```python
from build123d import *

# Parameters (mm, degrees)
F0_W      = 19
F0_H      = 30
F1_DEPTH  = 5
F3_DEPTH  = 3
F4_R      = 1
F4_R_2    = 0.895507
F5_DEPTH  = 25
F6_DEPTH  = 25
F7_W      = 43.592543
F7_H      = 48.578868
F8_DEPTH  = 2
F9_W      = 52.903849
F9_H      = 60.980772
F10_DEPTH = 1
F11_DEPTH = 25


with BuildPart() as f1:
    # F0 (on Front) → F1 (new body)
    with BuildSketch(Plane.XZ):
        Rectangle(F0_W, F0_H)
    extrude(amount=F1_DEPTH)

    # F2 (on face) → F3 (cut)
    with BuildSketch(Plane.XZ.offset(5)):
        with BuildLine():
            Line((-3, 0), (-3, -9))
            ThreePointArc((-3, -9), (0, -12), (3, -9))
            Line((3, -9), (3, 0))
            ThreePointArc((3, 0), (0, 2.961188), (-3, 0))
        make_face()
    extrude(amount=-F3_DEPTH, mode=Mode.SUBTRACT)

    # F4 (on face) → F5 (cut)
    with BuildSketch(Plane.XZ.offset(2)):
        with Locations((-6.5, 12)):
            Circle(F4_R)
        with Locations((6.5, 12)):
            Circle(F4_R)
        with Locations((6.5, -12)):
            Circle(F4_R)
        with Locations((-6.5, -12)):
            Circle(F4_R)
        with Locations((-6.5, 0)):
            Circle(F4_R)
        with Locations((6.5, 0)):
            Circle(F4_R_2)
    extrude(amount=-F5_DEPTH, mode=Mode.SUBTRACT)

    # F4 (on face) → F6 (cut)
    with BuildSketch(Plane.XZ.offset(2)):
        with Locations((-6.5, 12)):
            Circle(F4_R)
        with Locations((6.5, 12)):
            Circle(F4_R)
        with Locations((6.5, -12)):
            Circle(F4_R)
        with Locations((-6.5, -12)):
            Circle(F4_R)
        with Locations((-6.5, 0)):
            Circle(F4_R)
        with Locations((6.5, 0)):
            Circle(F4_R_2)
    extrude(amount=F6_DEPTH, mode=Mode.SUBTRACT)

    # F7 (on face) → F8 (cut)
    with BuildSketch(Plane.XZ.offset(5)):
        with Locations((0.917289, -2.192111)):
            Rectangle(F7_W, F7_H)
    extrude(amount=-F8_DEPTH, mode=Mode.SUBTRACT)

    # F9 (on face) → F10 (cut)
    with BuildSketch(Plane(origin=(0, 0, 0), x_dir=(-1, 0, 0), z_dir=(0, 1, 0))):
        with Locations((0.067309, -0.875001)):
            Rectangle(F9_W, F9_H)
    extrude(amount=-F10_DEPTH, mode=Mode.SUBTRACT)

    # F2 (on face) → F11 (cut)
    with BuildSketch(Plane.XZ.offset(5)):
        with BuildLine():
            Line((-3, 0), (-3, -9))
            ThreePointArc((-3, -9), (0, -12), (3, -9))
            Line((3, -9), (3, 0))
            ThreePointArc((3, 0), (0, 2.961188), (-3, 0))
        make_face()
    extrude(amount=-F11_DEPTH, mode=Mode.SUBTRACT)


solid = f1.part
```
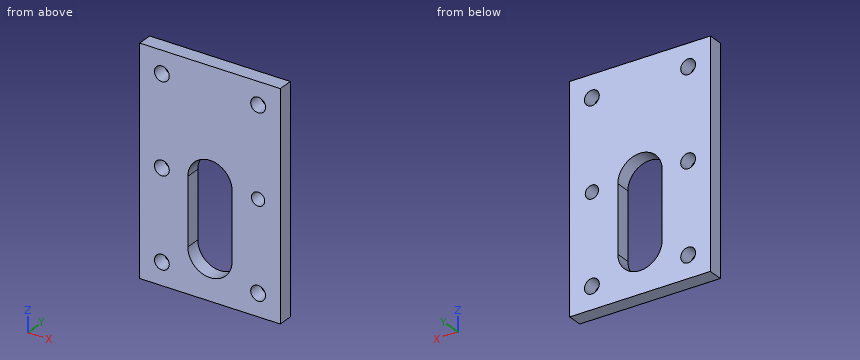
Geometry check sheet. Reference: the model listing, model coordinates, mm. Round coordinates to 2 decimals unless told otherwise and drop trailing zeros. Loops run counter-clockwise (first coordinate to the right, second up) from the corner with the lowest first, then second, coordinate; pieces in that order, holes last. Notation, with made-up numbers: M -39,31 L -23,31 A19 ccw -23,39 Z; hole C 67,-8.5 d8. An arc over 180 degrees is marked long. Return JSON: item names as keys, results as strings. Group by question number.
(1) Section check A-A, the plane z = -2. Enter the section's corners in (x, y), and give its area (3 significant figures).
(2) Scan lines: line 1 along Z through (x, y) = (-6.5, -1.45); line 2 along Z through (x, y) = (6.5, -1.85); line 3 along X through (y, z) = (-1.65, 0.5). Record each from-to range of solid material in increasing order. Write a range as [from, to].
(3) Section check C-C, the plane y = -1.3. Enter the section's corners in (x, z), and give its area (3 significant figures).
(4) Section check D-D, the plane x = 1.25. Enter the section's corners in (y, z).
(5) Section check B-B, the plane x = 6.5. Enter the section's corners in (y, z), and give its area (3 significant figures).
Data:
{
 "1": {"outline": "M -9.5,-3 L -3,-3 L -3,-1 L -9.5,-1 Z; M 3,-3 L 9.5,-3 L 9.5,-1 L 3,-1 Z", "area": "26.0 mm²"},
 "2": {"line 1": "[-15, -13], [-11, -1], [1, 11], [13, 15]", "line 2": "[-15, -13], [-11, -0.9], [0.9, 11], [13, 15]", "line 3": "[-9.5, -7.37], [-5.63, -2.95], [2.95, 5.76], [7.24, 9.5]"},
 "3": {"outline": "M -9.5,-15 L 9.5,-15 L 9.5,15 L -9.5,15 Z; hole C -6.5,-12 d2; hole C -6.5,0 d2; hole C -6.5,12 d2; hole M -3,-9 A3 ccw 3,-9 L 3,0 A3 ccw -3,0 Z; hole C 6.5,-12 d2; hole C 6.5,12 d2; hole C 6.5,0 d1.79", "area": "470 mm²"},
 "4": {"outline": "M -3,-15 L -1,-15 L -1,-11.73 L -3,-11.73 Z; M -3,2.69 L -1,2.69 L -1,15 L -3,15 Z"},
 "5": {"outline": "M -3,-15 L -1,-15 L -1,-13 L -3,-13 Z; M -3,-11 L -1,-11 L -1,-0.9 L -3,-0.9 Z; M -3,0.9 L -1,0.9 L -1,11 L -3,11 Z; M -3,13 L -1,13 L -1,15 L -3,15 Z", "area": "48.4 mm²"}
}
